from build123d import *

# Parameters (mm, degrees)
BOSS_EXTRUDE1_DEPTH = 63.5
SKETCH2_R           = 12.7
SKETCH2_R_2         = 1.5875
CUT_EXTRUDE1_DEPTH  = 3.175


with BuildPart() as part:
    # Sketch1 → Boss-Extrude1 (new body)
    with BuildSketch(Plane(origin=(0, 0, 0), x_dir=(0, 0, -1), z_dir=(1, 0, 0))):
        Polygon((-3.175, 0), (-50.8, 0), (-50.8, -3.175), (0, -3.175), (0, 0), (0, 47.625), (-3.175, 47.625), align=None)
    extrude(amount=BOSS_EXTRUDE1_DEPTH)

    # Sketch2 → Cut-Extrude1 (cut)
    with BuildSketch(Plane.XY.offset(3.175)):
        with Locations((31.75, 47.625)):
            Circle(SKETCH2_R)
        with Locations((12.7, 23.8125)):
            Circle(SKETCH2_R_2)
        with Locations((50.8, 23.8125)):
            Circle(SKETCH2_R_2)
    extrude(amount=-CUT_EXTRUDE1_DEPTH, mode=Mode.SUBTRACT)


solid = part.part
Part model, mm, in its own coordinate system. A direction names the side the tool comes from. Give positions to 0.01 mm unless a question says otherwise; leave off trailing zeros. Order: outer loops, then holes, each group sorted by start corner. A loop starts at its lowest first (then second) coordinate and runs counter-clockwise, first axis right, second up. Notation, with made-up numbers: (-1, 36.25) -> (24, 36.25) arc R10 cw to (24, 48.25) -> close; hole circle Ø4 at (32.5, -29). An arc over 180 degrees is marked (long way). Use one line per item in the form item = value.
(1) Tool access for faces 5 (the face through (9, 47.625, 2)), 6 (the face through (31, 24, 3.175)): list every direction of +Z, -Z, +X, -X, +Y, -Y with a clear straight run to the whole face (end or side of a thin tool).
Solution:
face_5 = +Z, -Z, +X, -X, +Y
face_6 = +Z, +X, -X, +Y
(2) Drill centre lines: line 1 (Y direction, x = 12.7, z = 2) (3 decimals); line 2 (Y direction, x = 16, z = 16.5) (3 decimals); line 3 (Y direction, x = 12, z = 2) (3 decimals). Where is each one in solid material? Low to high. Write a range as from..to.
Solution:
line_1 = -3.175..22.225, 25.4..47.625
line_2 = -3.175..0
line_3 = -3.175..22.388, 25.237..47.625
(3) Saw through at A-A (y = 41). Write the cut outline in (x, z) (3 decimals), then the cut area to 3 significant figures.
Solution:
outline = (0, 0) -> (20.915, 0) -> (20.915, 3.175) -> (0, 3.175) -> close; (42.585, 0) -> (63.5, 0) -> (63.5, 3.175) -> (42.585, 3.175) -> close
area = 133 mm²
(4) Saw through at B-B (x = 50.8). Write the cut outline in (y, z) (3 decimals).
Solution:
outline = (-3.175, 0) -> (22.225, 0) -> (22.225, 3.175) -> (0, 3.175) -> (0, 50.8) -> (-3.175, 50.8) -> close; (25.4, 0) -> (47.625, 0) -> (47.625, 3.175) -> (25.4, 3.175) -> close
(5) Flat gauge pins, fed straight in: P1, Ø24, axis at x = 43.5, z = 35, coming from the +Y side; P2, Ø24, axis at x = 23.5, y = 19.5, coming from the +Z side (3 decimals). Where does each tip first touch, or does it go through?
Solution:
P1 = 0
P2 = 3.175
(6) Saw through at C-C (x = 31.75). Write the cut outline in (y, z) (3 decimals).
Solution:
outline = (-3.175, 0) -> (34.925, 0) -> (34.925, 3.175) -> (0, 3.175) -> (0, 50.8) -> (-3.175, 50.8) -> close
(7) Saw through at D-D (z = 39.5). Write the cut outline in (x, y) (3 decimals), then the cut area to 3 significant figures.
Solution:
outline = (0, -3.175) -> (63.5, -3.175) -> (63.5, 0) -> (0, 0) -> close
area = 202 mm²
(8) Pull direction Y, two halves, no side cores. Call faces 1 (the face through (49.54, 22.85, 1.61)), 2 (the face through (0, -0.2, 14.2)), 3 (the face through (31, 0, 27)), 4 (the face through (13.433, 22.404, 1.61)): +Y half, -Y half, draft (parallel to the pull), parting line (faces both ways), or undercut.
Solution:
face_1 = undercut
face_2 = draft
face_3 = +Y half
face_4 = undercut
